```python
from build123d import *

# Parameters (mm, degrees)
SKETCH1_W               = 244.475
SKETCH1_H               = 244.475
MAIN_BODY_DEPTH         = 1.5875
SKETCH2_R               = 2.286
HINGES_LOCK_HOLES_DEPTH = 2.5875
SKETCH3_R               = 3.175
THREAD_HOLES_DEPTH      = 2.5875
SKETCH4_W               = 12.7
SKETCH4_H               = 12.7
LED_HOLES_DEPTH         = 2.5875


with BuildPart() as part:
    # Sketch1 → Main Body (new body)
    with BuildSketch(Plane(origin=(0, 0, 0), x_dir=(1, 0, 0), z_dir=(0, 1, 0))):
        with Locations((122.2375, 122.2375)):
            Rectangle(SKETCH1_W, SKETCH1_H)
    extrude(amount=MAIN_BODY_DEPTH)

    # Sketch2 → Hinges/Lock Holes (cut, through all)
    with BuildSketch(Plane(origin=(0, 1.5875, 0), x_dir=(1, 0, 0), z_dir=(0, 1, 0))):
        with Locations((54.1655, 235.6866)):
            Circle(SKETCH2_R)
        with Locations((71.4375, 235.6866)):
            Circle(SKETCH2_R)
        with Locations((173.0375, 235.6866)):
            Circle(SKETCH2_R)
        with Locations((190.3095, 235.6866)):
            Circle(SKETCH2_R)
        with Locations((74.4855, 9.906)):
            Circle(SKETCH2_R)
        with Locations((169.9895, 9.906)):
            Circle(SKETCH2_R)
    extrude(amount=-HINGES_LOCK_HOLES_DEPTH, mode=Mode.SUBTRACT)

    # Sketch3 → Thread Holes (cut, through all)
    with BuildSketch(Plane(origin=(0, 1.5875, 0), x_dir=(1, 0, 0), z_dir=(0, 1, 0))):
        with Locations((211.1375, 33.3375)):
            Circle(SKETCH3_R)
        with Locations((33.3375, 211.1375)):
            Circle(SKETCH3_R)
        with Locations((211.1375, 211.1375)):
            Circle(SKETCH3_R)
        with Locations((33.3375, 33.3375)):
            Circle(SKETCH3_R)
    extrude(amount=-THREAD_HOLES_DEPTH, mode=Mode.SUBTRACT)

    # Sketch4 → LED Holes (cut, through all)
    with BuildSketch(Plane(origin=(0, 1.5875, 0), x_dir=(1, 0, 0), z_dir=(0, 1, 0))):
        with Locations((122.2375, 25.4)):
            Rectangle(SKETCH4_W, SKETCH4_H)
        with Locations((25.4, 122.2375)):
            Rectangle(SKETCH4_W, SKETCH4_H)
        with Locations((122.2375, 219.075)):
            Rectangle(SKETCH4_W, SKETCH4_H)
        with Locations((219.075, 122.2375)):
            Rectangle(SKETCH4_W, SKETCH4_H)
    extrude(amount=-LED_HOLES_DEPTH, mode=Mode.SUBTRACT)


solid = part.part
```
CAD build for the part. Positions are in the model's coordinates, mm. Round coordinates to 2 decimals unless told otherwise and drop trailing zeros. Order: outer loops, then holes, each group sorted by start corner. A loop starts at its lowest first (then second) coordinate and runs counter-clockwise, first axis right, second up.
Item 1: Mould opens along Z. For faces 1 (the face through (121, 1.588, -124)), 2 (the face through (32.924, 0.805, -214.285)) say: pulls with the +Z half, pulls with the -Z half, needs draft (parallel to the pull), parting line crosses it, or undercut.
Item 2: Pin check, flat tip, straight feed: pin 1 (5.5 mm diameter, centred on x = 33.34, z = -33.34, fed in from +Y). Stop position of the tip, or through.
Item 3: Probe line 1 along Z through (x, y) = (217, 0.3) (1 decimal); line 2 along X through (y, z) = (0.3, -33) (3 decimals); line 3 along X through (y, z) = (1.1, -220.5) (1 decimal). List the from-to ranges inside material, lowest first.
Item 4: Saw through at B-B on x = 27. Write the cut outline in (y, z) (1 decimal), then the cut area to 3 significant figures.
Item 5: Saw through at A-A on x = 121. State how many separate pieces and enclosed holes the cut face has, then the cut area to 3 significant figures.
Reported:
1. face 1: needs draft
1. face 2: undercut
2. pin 1: passes through
3. line 1: z = -244.5 to -128.6, -115.9 to 0
3. line 2: x = 0 to 30.18, 36.495 to 207.98, 214.295 to 244.475
3. line 3: x = 0 to 115.9, 128.6 to 244.5
4. outline: (0, -244.5) - (1.6, -244.5) - (1.6, -128.6) - (0, -128.6) - close; (0, -115.9) - (1.6, -115.9) - (1.6, 0) - (0, 0) - close
4. area: 368 mm2
5. separate pieces: 3
5. enclosed holes: 0
5. area: 348 mm2
